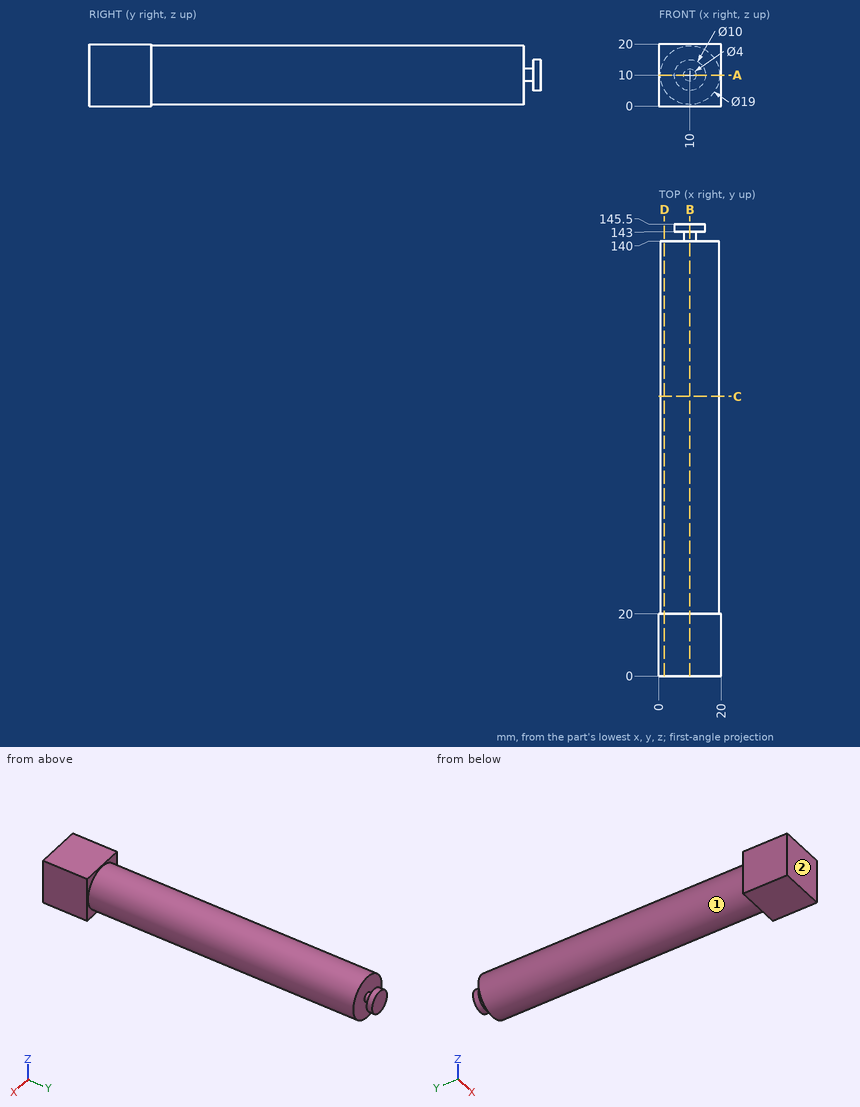
Input: dimensioned drawing with shaded views. Units: mm. Origin: part minimum x, y, z. A direction names the side the tool comes from. Round coordinates to 2 decimals unless told otherwise and drop trailing zeros. Loops run counter-clockwise (first coordinate to the right, second up) from the corner with the lowest first, then second, coordinate; pieces in that order, holes last. Notation, with made-up numbers: (24.25, -10) -> (48.25, -10) arc R13 ccw to (48.25, 9) -> close; hole circle Ø1 at (4, -13.75). An arc over 180 degrees is marked (long way). Answer as a JSON object with one key per item and string values. Group by question number.
1) Reachability of the marked faces 1 and 2 from +Z, -Z, +X, -X, +Y, -Y: full face, straight path, thin tool, end or side. Return the list, or none.
2) Section query C-C on y = 90. Output: boundary loops of the cut face in (x, z), plus the area to 3 significant figures.
3) Ray query, L1, parallel to Y at x = 4.25, z = 4; L2, parallel to Y at x = 7.75, z = 7.25; L3, parallel to X at y = 56, z = 10. Return the intervals inside material, ascending.
4) Pin query (flat end, axial travel): pin 1 (6 mm diameter, centred on y = 53.5, z = 10.5, fed in from +X); pin 2 (4 mm diameter, centred on x = 11, y = 81, fed in from +Z); pin 3 (6 mm diameter, centred on x = 14, z = 10.5, fed in from -Y); pin 4 (1.5 mm diameter, centred on x = 3, y = 58.5, fed in from +Z). Return the tip coordinate at first contact, or that it passes through.
5) Section query B-B on x = 10. Output: boundary loops of the cut face in (y, z).
6) Section query A-A on z = 10. Output: boundary loops of the cut face in (x, y).
7) Section query D-D on x = 1.75. Output: boundary loops of the cut face in (y, z).
Reply:
{
 "1": {"face 1": "+Y", "face 2": "+Z, -Z, +X, -X, -Y"},
 "2": {"outline": "circle Ø19 at (10, 10)", "area": "284 mm2"},
 "3": {"L1": "y = 0 to 140", "L2": "y = 0 to 140, 143 to 145.5", "L3": "x = 0.5 to 19.5"},
 "4": {"pin 1": "stops at x = 19.5", "pin 2": "stops at z = 19.5", "pin 3": "stops at y = 0", "pin 4": "stops at z = 17.15"},
 "5": {"outline": "(0, 0) -> (20, 0) -> (20, 0.5) -> (140, 0.5) -> (140, 8) -> (143, 8) -> (143, 5) -> (145.5, 5) -> (145.5, 15) -> (143, 15) -> (143, 12) -> (140, 12) -> (140, 19.5) -> (20, 19.5) -> (20, 20) -> (0, 20) -> close"},
 "6": {"outline": "(0, 0) -> (20, 0) -> (20, 20) -> (19.5, 20) -> (19.5, 140) -> (12, 140) -> (12, 143) -> (15, 143) -> (15, 145.5) -> (5, 145.5) -> (5, 143) -> (8, 143) -> (8, 140) -> (0.5, 140) -> (0.5, 20) -> (0, 20) -> close"},
 "7": {"outline": "(0, 0) -> (20, 0) -> (20, 5.29) -> (140, 5.29) -> (140, 14.71) -> (20, 14.71) -> (20, 20) -> (0, 20) -> close"}
}
